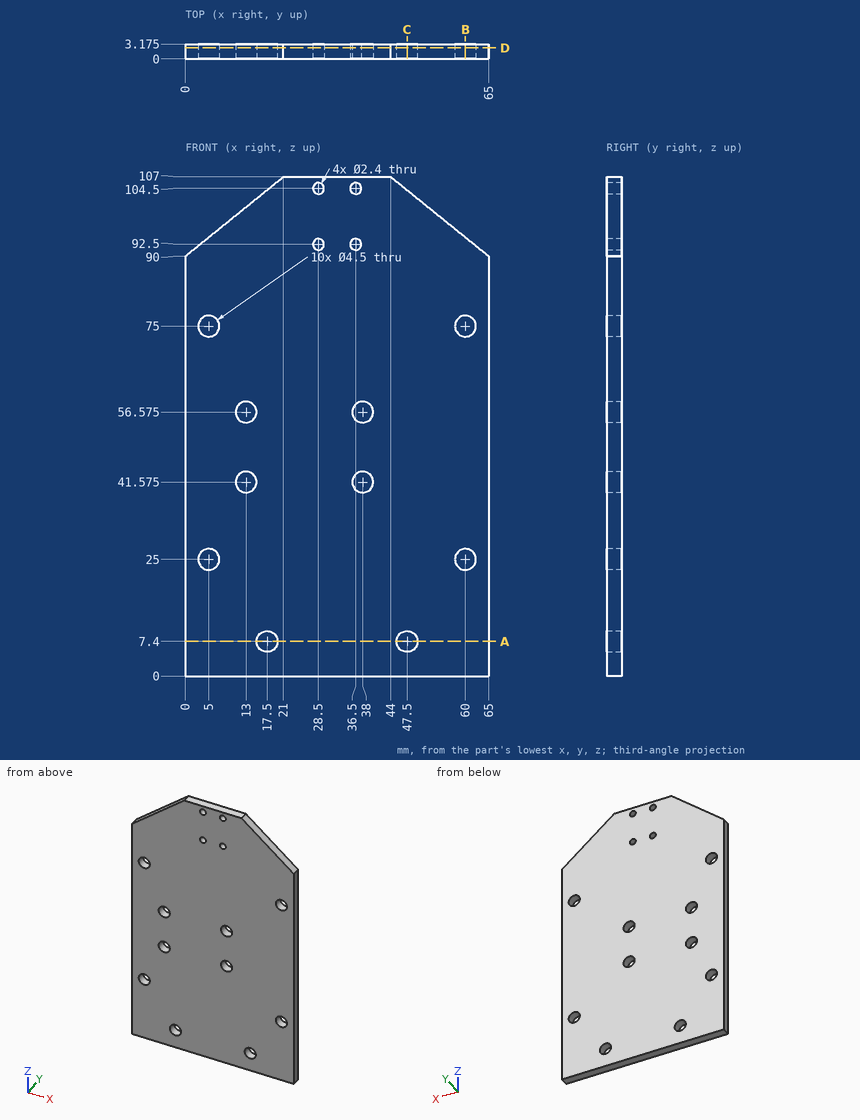
Could you check a few things on this drawing? It's one solid part, dimensions in mm from its lowest x, y, z. Coordinates: 2 decimals unless noted, no trailing zeros. Order: outer loops, then holes, each group sorted by start corner. A loop starts at its lowest first (then second) coordinate and runs counter-clockwise, first axis right, second up. Notation, with made-up numbers: (-7, -35.75) - (34, -35.75) arc R30 cw to (34, -7.75) - close; hole circle Ø2 at (-3.5, -1.75). An arc over 180 degrees is marked (long way). Answer as a JSON object with one key per item and string values. Group by question number.
Q1. Imagine slicing it at D-D (y = 2.35). Give the number of separate pieces and of enclosed holes in the cut face, and give its area (3 significant figures).
Q2. Will this pin go through, and if not, where does the flat tip stop? P1, Ø6, axis at x = 17.5, z = 7.4, coming from the -Y side.
Q3. Imagine slicing it at C-C (x = 47.5). Please give me the cut outline in (y, z) (3 decimals).
Q4. I need wall thicknesses on line 1 (X direction, y = 2.2, z = 75); line 2 (X direction, y = 1, z = 7.4); line 3 (Z direction, x = 28.5, y = 2). Which ranges of each line are inside material? Lowest first, please. Write a range as from..to.
Q5. Imagine slicing it at B-B (x = 60). Please give me the cut outline in (y, z) (3 decimals).
Q6. Imagine slicing it at A-A (z = 7.4). Please give me the cut outline in (x, y) (3 decimals).
Determined:
{
 "1": {"separate pieces": "1", "enclosed holes": "14", "area": "6,420 mm2"},
 "2": {"P1": "stops at y = 0"},
 "3": {"outline": "(0, 0) - (3.175, 0) - (3.175, 5.15) - (0, 5.15) - close; (0, 9.65) - (3.175, 9.65) - (3.175, 104.167) - (0, 104.167) - close"},
 "4": {"line 1": "x = 0..2.75, 7.25..57.75, 62.25..65", "line 2": "x = 0..15.25, 19.75..45.25, 49.75..65", "line 3": "z = 0..91.3, 93.7..103.3, 105.7..107"},
 "5": {"outline": "(0, 0) - (3.175, 0) - (3.175, 22.75) - (0, 22.75) - close; (0, 27.25) - (3.175, 27.25) - (3.175, 72.75) - (0, 72.75) - close; (0, 77.25) - (3.175, 77.25) - (3.175, 94.048) - (0, 94.048) - close"},
 "6": {"outline": "(0, 0) - (15.25, 0) - (15.25, 3.175) - (0, 3.175) - close; (19.75, 0) - (45.25, 0) - (45.25, 3.175) - (19.75, 3.175) - close; (49.75, 0) - (65, 0) - (65, 3.175) - (49.75, 3.175) - close"}
}
